from build123d import *

# Parameters (mm, degrees)
F1_DEPTH = 2.9972


with BuildPart() as f1:
    # F0 (on Right) → F1 (new body, symmetric)
    with BuildSketch(Plane.YZ):
        with BuildLine():
            Line((0, 50.8), (0, 0))
            Line((0, 0), (19.05, 0))
            ThreePointArc((19.05, 0), (23.5401280605, 1.8598719395), (25.4, 6.35))
            Line((25.4, 6.35), (25.4, 12.7))
            ThreePointArc((25.4, 12.7), (27.2598719395, 17.1901280605), (31.75, 19.05))
            Line((31.75, 19.05), (57.15, 19.05))
            Line((57.15, 19.05), (57.15, 25.4))
            Line((57.15, 25.4), (50.8, 25.4))
            Line((50.8, 25.4), (50.8, 50.8))
            Line((50.8, 50.8), (0, 50.8))
        make_face()
    extrude(amount=F1_DEPTH, both=True)


solid = f1.part
For this review, take the finished solid that the model builds, in its own axes (mm). A direction names the side the tool comes from. Coordinates: 2 decimals unless noted, no trailing zeros. Order: outer loops, then holes, each group sorted by start corner. A loop starts at its lowest first (then second) coordinate and runs counter-clockwise, first axis right, second up. Notation, with made-up numbers: (0.25, -39) - (47.25, -39) arc R17 ccw to (47.25, -21) - close; hole circle Ø7 at (23.25, 58). An arc over 180 degrees is marked (long way). Answer as CSV lines item,"result". Start each with the question number.
1) To check wall thickness, follow line 1 along Y through (x, z) = (1.25, 7); line 2 along Y through (x, z) = (-2.5, 40.5); line 3 along Z through (x, y) = (-0.65, 43.5). State the ranges of each line that lie inside material, in increasing order. Write a range as [from, to].
2) Add section B-B (z = 7.5). State the section outline as (x, y) points, then the cut area to 3 significant figures.
3) Insertion check: P1, Ø2, axis at x = 0.5, y = 40, coming from the -Z side; P2, Ø1.8, axis at x = -1.5, y = 55, coming from the +Z side; P3, Ø1.8, axis at x = -1.5, z = 40.5, coming from the +Y side. Each pin has a flat end and moves straight along its axis. Give the tip position at first contact, or say it passes through.
4) Draft analysis for pull direction Z (two halves, no side actions). For faces 4 (the cylindrical face through (0.04, 23.49, 1.81)), 5 (the flat face through (0, 57.15, 22)), 6 (the flat face through (0, 54, 25.4)), state which applies: +Z half, -Z half, draft (parallel to the pull), parting line (faces both ways), or undercut.
5) Machinability: for faces 1 (the flat face through (0, 44, 19.05)), 2 (the flat face through (2.997, 22, 31)), 3 (the flat face through (0, 50.8, 38)), which of the approach directions +Z, -Z, +X, -X, +Y, -Y give a long, thin tool a straight path to every point of the face, cutting with its end or side? Answer none if there is none.
6) Add section C-C (y = 33.5). State the section outline as (x, z) points.
7) Add section A-A (x = 0.15). State the section outline as (y, z) points.
Result:
1,line 1,"[0, 25.4]"
1,line 2,"[0, 50.8]"
1,line 3,"[19.05, 50.8]"
2,outline,"(-3, 0) - (3, 0) - (3, 25.4) - (-3, 25.4) - close"
2,area,"152 mm^2"
3,P1,"z = 19.05"
3,P2,"z = 25.4"
3,P3,"y = 50.8"
4,face 4,"-Z half"
4,face 5,"draft"
4,face 6,"+Z half"
5,face 1,"-Z, +X, -X, +Y"
5,face 2,"+Z, -Z, +X, +Y, -Y"
5,face 3,"+Z, +X, -X, +Y"
6,outline,"(-3, 19.05) - (3, 19.05) - (3, 50.8) - (-3, 50.8) - close"
7,outline,"(0, 0) - (19.05, 0) arc R6.35 ccw to (25.4, 6.35) - (25.4, 12.7) arc R6.35 cw to (31.75, 19.05) - (57.15, 19.05) - (57.15, 25.4) - (50.8, 25.4) - (50.8, 50.8) - (0, 50.8) - close"
